```python
from build123d import *

# Parameters (mm, degrees)
SKETCH1_R           = 0.45
SKETCH1_R_2         = 3.5
SKETCH1_R_3         = 2.3
SKETCH1_R_4         = 1.2
BOSS_EXTRUDE1_DEPTH = 1.5
BOSS_EXTRUDE2_START = 1.5
SKETCH1_4_R         = 3.5
SKETCH1_4_R_2       = 2.3
BOSS_EXTRUDE2_DEPTH = 2.5
SKETCH1_5_R         = 2.3
SKETCH1_5_R_2       = 1.2
CUT_EXTRUDE1_DEPTH  = 0.5


with BuildPart() as part:
    # Sketch1 → Boss-Extrude1 (new body)
    # profile 1 of 4: a face of its own
    with BuildSketch(Plane(origin=(0, 0, 0), x_dir=(1, 0, 0), z_dir=(0, 1, 0))):
        with BuildLine():
            ThreePointArc((-1.959591794, -2.9), (-3.5, 0), (-1.959591794, 2.9))
            Line((-1.959591794, 2.9), (-14.5, 1.5))
            ThreePointArc((-14.5, 1.5), (-16, 0), (-14.5, -1.5))
            Line((-14.5, -1.5), (-1.959591794, -2.9))
        make_face()
        with Locations(Location((-14.5, 0, 0), (0, 0, 270))):
            Circle(SKETCH1_R, mode=Mode.SUBTRACT)
        with Locations(Location((-12.5, 0, 0), (0, 0, 270))):
            Circle(SKETCH1_R, mode=Mode.SUBTRACT)
        with Locations(Location((-10.5, 0, 0), (0, 0, 270))):
            Circle(SKETCH1_R, mode=Mode.SUBTRACT)
        with Locations(Location((-8.5, 0, 0), (0, 0, 270))):
            Circle(SKETCH1_R, mode=Mode.SUBTRACT)
        with Locations(Location((-6.5, 0, 0), (0, 0, 270))):
            Circle(SKETCH1_R, mode=Mode.SUBTRACT)
        with Locations(Location((-4.5, 0, 0), (0, 0, 270))):
            Circle(SKETCH1_R, mode=Mode.SUBTRACT)
    # profile 2 of 4: a face of its own
    with BuildSketch(Plane(origin=(0, 0, 0), x_dir=(1, 0, 0), z_dir=(0, 1, 0))):
        with BuildLine():
            Line((14.5, 1.5), (1.959591794, 2.9))
            ThreePointArc((1.959591794, 2.9), (3.091000751, 1.641863076), (3.5, 0))
            ThreePointArc((3.5, 0), (3.091000751, -1.641863076), (1.959591794, -2.9))
            Line((1.959591794, -2.9), (14.5, -1.5))
            ThreePointArc((14.5, -1.5), (16, 0), (14.5, 1.5))
        make_face()
        with Locations(Location((4.5, 0, 0), (0, 0, 270))):
            Circle(SKETCH1_R, mode=Mode.SUBTRACT)
        with Locations(Location((6.5, 0, 0), (0, 0, 270))):
            Circle(SKETCH1_R, mode=Mode.SUBTRACT)
        with Locations(Location((8.5, 0, 0), (0, 0, 270))):
            Circle(SKETCH1_R, mode=Mode.SUBTRACT)
        with Locations(Location((10.5, 0, 0), (0, 0, 270))):
            Circle(SKETCH1_R, mode=Mode.SUBTRACT)
        with Locations(Location((12.5, 0, 0), (0, 0, 270))):
            Circle(SKETCH1_R, mode=Mode.SUBTRACT)
        with Locations(Location((14.5, 0, 0), (0, 0, 270))):
            Circle(SKETCH1_R, mode=Mode.SUBTRACT)
    # profile 3 of 4: a face of its own
    with BuildSketch(Plane(origin=(0, 0, 0), x_dir=(1, 0, 0), z_dir=(0, 1, 0))):
        Circle(SKETCH1_R_2)
        Circle(SKETCH1_R_3, mode=Mode.SUBTRACT)
    # profile 4 of 4: a face of its own
    with BuildSketch(Plane(origin=(0, 0, 0), x_dir=(1, 0, 0), z_dir=(0, 1, 0))):
        Circle(SKETCH1_R_3)
        with Locations(Location((0, 0, 0), (0, 0, 270))):
            Circle(SKETCH1_R_4, mode=Mode.SUBTRACT)
    extrude(amount=BOSS_EXTRUDE1_DEPTH)

    # Sketch1<4> → Boss-Extrude2 (add)
    with BuildSketch(Plane(origin=(0, 0, 0), x_dir=(1, 0, 0), z_dir=(0, 1, 0)).offset(BOSS_EXTRUDE2_START)):
        with Locations(Location((0, 0, 0), (0, 0, 124.04773237))):
            Circle(SKETCH1_4_R)
        with Locations(Location((0, 0, 0), (0, 0, 270))):
            Circle(SKETCH1_4_R_2, mode=Mode.SUBTRACT)
    extrude(amount=BOSS_EXTRUDE2_DEPTH)

    # Sketch1<5> → Cut-Extrude1 (cut)
    with BuildSketch(Plane(origin=(0, 0, 0), x_dir=(1, 0, 0), z_dir=(0, 1, 0))):
        with Locations(Location((0, 0, 0), (0, 0, 270))):
            Circle(SKETCH1_5_R)
        with Locations(Location((0, 0, 0), (0, 0, 270))):
            Circle(SKETCH1_5_R_2, mode=Mode.SUBTRACT)
    extrude(amount=CUT_EXTRUDE1_DEPTH, mode=Mode.SUBTRACT)


solid = part.part
```
Build history of the part. All positions in model axes, mm. A direction names the side the tool comes from. Give positions to 0.01 mm unless a question says otherwise; leave off trailing zeros. Loops run counter-clockwise (first coordinate to the right, second up) from the corner with the lowest first, then second, coordinate; pieces in that order, holes last.
1) Probe line 1 along Y through (x, z) = (3.5, -1); line 2 along X through (y, z) = (2.6, -0.25); line 3 along X through (y, z) = (2.7, 1). List the from-to ranges inside material, lowest first.
Values follow:
line 1: y = 0 to 1.5
line 2: x = -3.49 to -2.29, 2.29 to 3.49
line 3: x = -3.35 to -2.07, 2.07 to 3.35
2) Two-plate mould, pull along Z, no slides. Class faces 4 (the face through (16, 1, 0)), 5 (the face through (2.4, 4, -0.6)), 6 (the face through (-14.94, 0.74, -0.1)), 7 (the face through (0.691, 0.246, 2.194)): released by +Z, released by -Z, zero draft, split by the parting line, or undercut.
Values follow:
face 4: split by the parting line
face 5: zero draft
face 6: undercut
face 7: undercut
3) Band-saw the part on B-B on y = 3.5. List the corners of the cut face in (x, z), then the cut area to 3 significant figures.
Values follow:
outline: circle Ø7 at (0, 0); hole circle Ø4.6 at (0, 0)
area: 21.9 mm2
4) Band-saw the part on D-D on z = -2. List the corners of the cut face in (x, y), then the cut area to 3 significant figures.
Values follow:
outline: (-10.02, 0) - (-1.14, 0) - (-1.14, 0.5) - (1.14, 0.5) - (1.14, 0) - (10.02, 0) - (10.02, 1.5) - (2.87, 1.5) - (2.87, 4) - (1.14, 4) - (1.14, 1.5) - (-1.14, 1.5) - (-1.14, 4) - (-2.87, 4) - (-2.87, 1.5) - (-10.02, 1.5) - close
area: 37.6 mm2
5) Band-saw the part on A-A on x = 4.5. List the corners of the cut face in (y, z), then the cut area to 3 significant figures.
Values follow:
outline: (0, -2.62) - (1.5, -2.62) - (1.5, -0.45) - (0, -0.45) - close; (0, 0.45) - (1.5, 0.45) - (1.5, 2.62) - (0, 2.62) - close
area: 6.50 mm2
6) Band-saw the part on C-C on x = -6.5. List the corners of the cut face in (y, z).
Values follow:
outline: (0, -2.39) - (1.5, -2.39) - (1.5, -0.45) - (0, -0.45) - close; (0, 0.45) - (1.5, 0.45) - (1.5, 2.39) - (0, 2.39) - close
7) 3-axis set-ups, long thin cutter, end or side, ignore diameter. For faces 1 (the face through (0.691, 2.732, 2.194)), 2 (the face through (-1, 0.5, 1)), 3 (the face through (-16, 1, 0)): which of +Z, -Z, +X, -X, +Y, -Y reach the whole face in a straight line?
Values follow:
face 1: +Y
face 2: -Y
face 3: -X, +Y, -Y
8) Drop flat-ended pins along their axis: P1, Ø1.9, axis at x = 0, z = 0, coming from the +Y side; P2, Ø3, axis at x = -7.5, z = -1.5, coming from the +Y side; P3, Ø1, axis at y = 3.5, z = -0.5, coming from the +X side. Give the stop position or say it passes through.
Values follow:
P1: passes through
P2: stops at y = 1.5
P3: stops at x = 3.5
